The figure shows three views and two pictorial views of one solid part (mm, origin at its lowest corner). Answer the questions. A direction names the side the tool comes from. Give positions to 0.01 mm unless a question says otherwise; leave off trailing zeros. Order: outer loops, then holes, each group sorted by start corner. A loop starts at its lowest first (then second) coordinate and runs counter-clockwise, first axis right, second up. Notation, with made-up numbers: (25, 75.25) - (51, 75.25) arc R30 ccw to (51, 103.25) - close; hole circle Ø5 at (-12.75, 25.25). An arc over 180 degrees is marked (long way). Answer as CSV lines item,"result". Start each with the question number.
1. Consider line 1 along X through (y, z) = (3.5, 14.75); line 2 along Y through (x, z) = (1.25, 13.75); line 3 along X through (y, z) = (1.75, 11). Determine where each line is inside the solid, lowest interval first. Write a range as [from, to].
2. Section B-B on z = 14.75 is taken. Give the vertices of the cut face in (x, y).
3. A flat-ended cylindrical pin translates along its axis: pin 1 (3 mm diameter, centred on x = 1.5, z = 5.5, fed in from -Y). Find the tip coordinate at first contact, or state that the pin passes through.
4. Which of the six approach directions +Z, -Z, +X, -X, +Y, -Y give full straight-line access (tool end or side, diameter ignored) to the marked faces 1 and 2?
5. Section A-A on z = 20 is taken. Give the vertices of the cut face in (x, y), and give its area (3 significant figures).
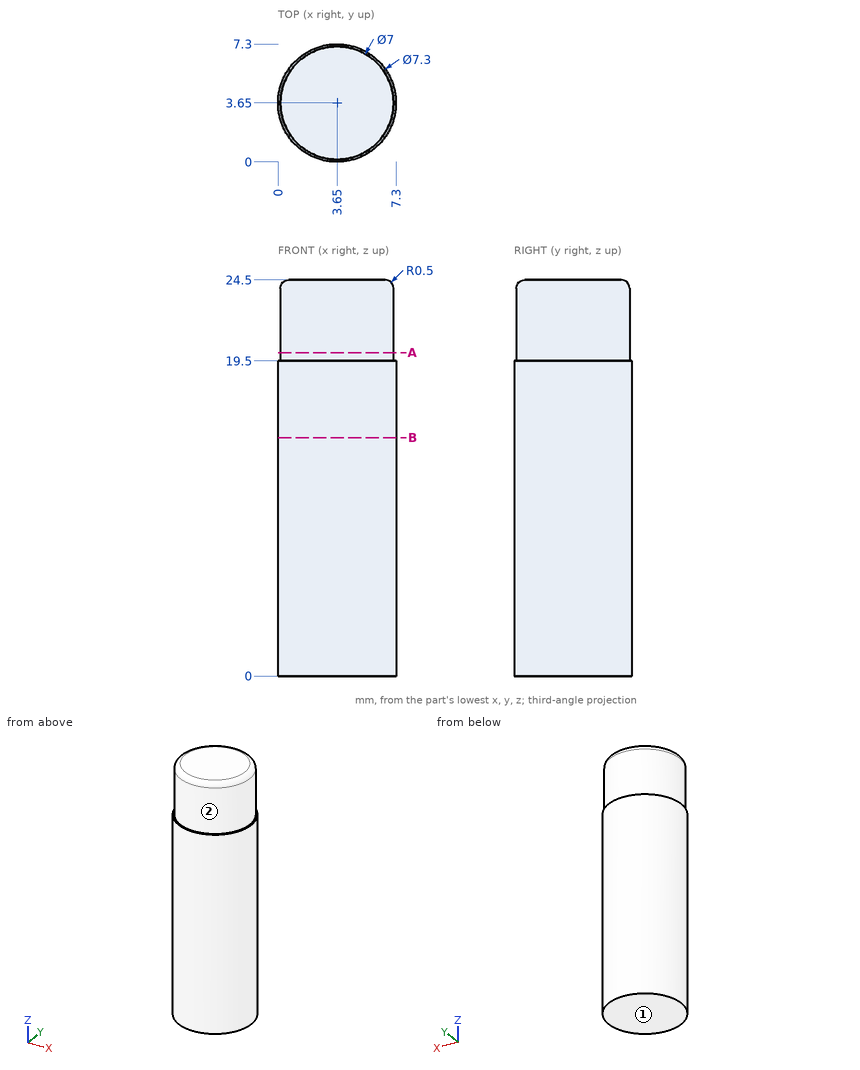
Checks:
1,line 1,"x = [0, 7.3]"
1,line 2,"y = [0.9, 6.4]"
1,line 3,"x = [0.53, 6.77]"
2,outline,"circle Ø7.3 at (3.65, 3.65)"
3,pin 1,"stops at y = 0.06"
4,face 1,"-Z, +X, -X, +Y, -Y"
4,face 2,"+Z"
5,outline,"circle Ø7 at (3.65, 3.65)"
5,area,"38.5 mm²"
